Check sheet for the modelled part. Datum: model origin and axes. Units: mm. Face numbers are marked on the shaded views. A direction names the side the tool comes from. Coordinates: 2 decimals unless noted, no trailing zeros. Order: outer loops, then holes, each group sorted by start corner. A loop starts at its lowest first (then second) coordinate and runs counter-clockwise, first axis right, second up.
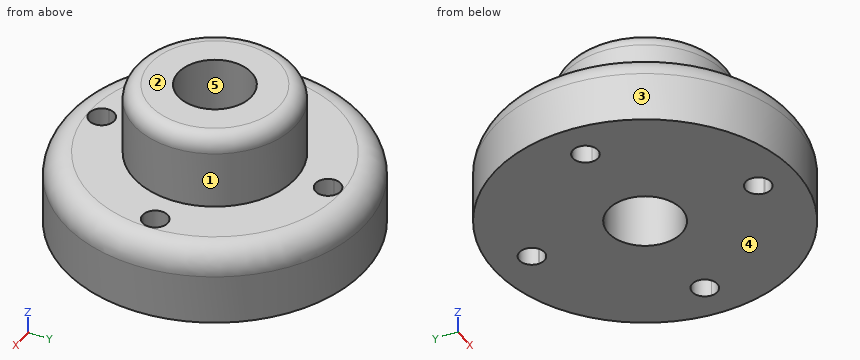
from build123d import *

# Parameters (mm, degrees)
F0_R     = 30
F0_R_2   = 16.1
F1_DEPTH = 14.9
F0_R_3   = 7.315
F2_DEPTH = 29.5
F3_R     = 5
F4_R     = 3.2


with BuildPart() as f1:
    # F0 (on Top) → F1 (new body)
    with BuildSketch(Plane.XY):
        Circle(F0_R)
        with BuildLine():
            ThreePointArc((-22.159865, -2.496069), (-24.8, 0), (-22.159865, 2.496069))
            ThreePointArc((-22.159865, 2.496069), (-15.768481, 15.768481), (-2.496069, 22.159865))
            ThreePointArc((-2.496069, 22.159865), (-0.070095, 24.799017), (2.5, 22.3))
            ThreePointArc((2.5, 22.3), (2.499017, 22.229905), (2.496069, 22.159865))
            ThreePointArc((2.496069, 22.159865), (15.768481, 15.768481), (22.159865, 2.496069))
            ThreePointArc((22.159865, 2.496069), (24.017507, 1.816636), (24.8, 0))
            ThreePointArc((24.8, 0), (24.017507, -1.816636), (22.159865, -2.496069))
            ThreePointArc((22.159865, -2.496069), (15.768481, -15.768481), (2.496069, -22.159865))
            ThreePointArc((2.496069, -22.159865), (2.499017, -22.229905), (2.5, -22.3))
            ThreePointArc((2.5, -22.3), (-0.070095, -24.799017), (-2.496069, -22.159865))
            ThreePointArc((-2.496069, -22.159865), (-15.768481, -15.768481), (-22.159865, -2.496069))
        make_face(mode=Mode.SUBTRACT)
        with BuildLine():
            ThreePointArc((-22.159865, 2.496069), (-20.483364, 1.717507), (-19.8, 0))
            ThreePointArc((-19.8, 0), (-20.483364, -1.717507), (-22.159865, -2.496069))
            ThreePointArc((-22.159865, -2.496069), (-15.768481, -15.768481), (-2.496069, -22.159865))
            ThreePointArc((-2.496069, -22.159865), (0, -19.8), (2.496069, -22.159865))
            ThreePointArc((2.496069, -22.159865), (15.768481, -15.768481), (22.159865, -2.496069))
            ThreePointArc((22.159865, -2.496069), (19.8, 0), (22.159865, 2.496069))
            ThreePointArc((22.159865, 2.496069), (15.768481, 15.768481), (2.496069, 22.159865))
            ThreePointArc((2.496069, 22.159865), (0, 19.8), (-2.496069, 22.159865))
            ThreePointArc((-2.496069, 22.159865), (-15.768481, 15.768481), (-22.159865, 2.496069))
        make_face()
        Circle(F0_R_2, mode=Mode.SUBTRACT)
    extrude(amount=F1_DEPTH)

    # F0 (on Top) → F2 (join)
    with BuildSketch(Plane.XY):
        Circle(F0_R_2)
        Circle(F0_R_3, mode=Mode.SUBTRACT)
    extrude(amount=F2_DEPTH)

    # F3
    f3_edges = [f1.edges().sort_by_distance(p)[0] for p in [
        (-30, 0, 14.9),
    ]]
    fillet(f3_edges, radius=F3_R)

    # F4
    f4_edges = [f1.edges().sort_by_distance(p)[0] for p in [
        (-16.1, 0, 29.5),
    ]]
    fillet(f4_edges, radius=F4_R)


solid = f1.part
(1) Thickness scan on probe 1 along Y at (x, z) = (0, 9.75) (3 decimals); probe 2 along Y at (x, z) = (0, 23.25) (3 decimals); probe 3 along Y at (x, z) = (0, 11) (1 decimal). Record the ranges inside material, lowest first.
Filled in:
probe 1: y = -30 to -24.8, -19.8 to -7.315, 7.315 to 19.8, 24.8 to 30
probe 2: y = -16.1 to -7.315, 7.315 to 16.1
probe 3: y = -29.9 to -24.8, -19.8 to -7.3, 7.3 to 19.8, 24.8 to 29.9
(2) Cross-section at B-B (z = 11.25). Enter the section's corners in (x, y) (3 decimals).
Filled in:
outline: circle Ø59.629 at (0, 0); hole (-22.16, -2.496) arc R2.5 ccw to (-19.8, 0) arc R2.5 ccw to (-22.16, 2.496) arc R2.5 ccw (long way) to start; hole circle Ø14.63 at (0, 0); hole (2.496, -22.16) arc R2.5 ccw (long way) to (2.5, -22.3) arc R2.5 ccw to start; hole (2.496, 22.16) arc R2.5 ccw to (2.5, 22.3) arc R2.5 ccw (long way) to start; hole (22.16, -2.496) arc R2.5 ccw to (24.8, 0) arc R2.5 ccw to (22.16, 2.496) arc R2.5 ccw to start
(3) Tool access check on the marked faces 1 and 2. Record the directions out of +Z, -Z, +X, -X, +Y, -Y that give a thin tool (end or side, any length) a straight path to the whole face; none if there is none.
Filled in:
face 1: +Z
face 2: +Z, +X, -X, +Y, -Y
(4) Cross-section at A-A (x = 0). Enter the section's corners in (y, z) (3 decimals).
Filled in:
outline: (-30, 0) - (-24.8, 0) - (-24.8, 14.9) - (-25, 14.9) arc R5 ccw to (-30, 9.9) - close; (-19.8, 0) - (-7.315, 0) - (-7.315, 29.5) - (-12.9, 29.5) arc R3.2 ccw to (-16.1, 26.3) - (-16.1, 14.9) - (-19.8, 14.9) - close; (7.315, 0) - (19.8, 0) - (19.8, 14.9) - (16.1, 14.9) - (16.1, 26.3) arc R3.2 ccw to (12.9, 29.5) - (7.315, 29.5) - close; (24.8, 0) - (30, 0) - (30, 9.9) arc R5 ccw to (25, 14.9) - (24.8, 14.9) - close
(5) Cross-section at C-C (z = 23.25). Enter the section's corners in (x, y) (3 decimals).
Filled in:
outline: circle Ø32.2 at (0, 0); hole circle Ø14.63 at (0, 0)
(6) Release check for a two-part mould opening along Y. For the marked faces 3, 4 and 5 record: +Y half, -Y half, draft (parallel to the pull), parting line (faces both ways), or undercut.
Filled in:
face 3: parting line
face 4: draft
face 5: undercut
(7) Go/stop test with flat-tipped pins: P1, Ø4, axis at x = 7, z = 21, coming from the +Y side; P2, Ø6, axis at x = -16.5, z = 10.5, coming from the +Y side; P3, Ø12, axis at y = -6, z = 14.5, coming from the +X side; P4, Ø4, axis at x = -2, y = 16, coming from the -Z side. Record where each tip stops, or that it passes through.
Filled in:
P1: stops at y = 15.3
P2: stops at y = 26.77
P3: stops at x = 29.94
P4: stops at z = 0
